```python
from build123d import *

# Parameters (mm, degrees)
SKETCH1_R           = 12.0269
BOSS_EXTRUDE1_DEPTH = 3.03784
BOSS_EXTRUDE2_DEPTH = 5.0038
FILLET1_R           = 5.08
FILLET2_R           = 0.381


with BuildPart() as part:
    # Sketch1 → Boss-Extrude1 (new body)
    with BuildSketch(Plane(origin=(0, 0, 0), x_dir=(1, 0, 0), z_dir=(0, 1, 0))):
        with Locations(Location((0, 0, 0), (0, 0, 270))):
            Circle(SKETCH1_R)
        with BuildLine():
            Line((-3.334475635, 5.1562), (3.334475635, 5.1562))
            ThreePointArc((3.334475635, 5.1562), (6.14045, 0), (3.334475635, -5.1562))
            Line((3.334475635, -5.1562), (-3.334475635, -5.1562))
            ThreePointArc((-3.334475635, -5.1562), (-6.14045, 0), (-3.334475635, 5.1562))
        make_face(mode=Mode.SUBTRACT)
    extrude(amount=BOSS_EXTRUDE1_DEPTH)

    # Sketch3 → Boss-Extrude2 (add, symmetric)
    with BuildSketch(Plane.XY):
        Polygon((-6.14045, 3.03784), (-13.285214528, 3.03784), (-17.255205114, -0.932150585), (-15.10712785, -3.08022785), (-12.0269, 0), (-6.14045, 0), align=None)
    extrude(amount=BOSS_EXTRUDE2_DEPTH, both=True)

    # Fillet1
    fillet1_edges = [part.edges().sort_by_distance(p)[0] for p in [
        (-13.285214528, 3.03784, 0),
    ]]
    fillet(fillet1_edges, radius=FILLET1_R)

    # Fillet2
    fillet2_edges = [part.edges().sort_by_distance(p)[0] for p in [
        (6.14045, 3.03784, 0),
        (0, 3.03784, -5.1562),
        (12.0269, 3.03784, 0),
        (-10.936558379, 1.51892, -5.0038),
        (-10.936558379, 1.51892, 5.0038),
        (-11.058784005, 3.03784, 5.0038),
        (-16.181166482, -2.006189217, 5.0038),
        (-11.058784005, 3.03784, -5.0038),
        (-16.181166482, -2.006189217, -5.0038),
        (-17.255205114, -0.932150585, 0),
        (-16.014158597, 0.308895932, -5.0038),
        (-16.014158597, 0.308895932, 5.0038),
        (-13.125041468, 2.651148025, -5.0038),
        (-13.125041468, 2.651148025, 5.0038),
        (-6.14045, 3.03784, 0),
        (0, 3.03784, 5.1562),
    ]]
    fillet(fillet2_edges, radius=FILLET2_R)


solid = part.part
```
Read the model definition and answer for the solid it produces. Units are mm, in the model's axes. A direction names the side the tool comes from. Give positions to 0.01 mm unless a question says otherwise; leave off trailing zeros. Write each loop counter-clockwise with the first axis right and the second up, starting at its lowest first coordinate (ties: lowest second). Pieces come first, ordered by that corner, then holes. Notation, with made-up numbers: (-5.5, 32) -> (24.5, 32) arc R21 ccw to (24.5, 36) -> close; hole circle Ø5 at (51.5, 37). An arc over 180 degrees is marked (long way). Answer in a Markdown table with one row per item.
1) Determine the mould class of faces 6 (the cylindrical face through (-6.14, 1.31, 0.09)), 7 (the flat face through (-13.589, -1.562, 0.07)), 8 (the cylindrical face through (-15.82, 0.35, -4.89)) for opening direction Z: released by +Z, released by -Z, zero draft, split by the parting line, or undercut.
Results list:
| item | result |
|---|---|
| face 6 | undercut |
| face 7 | zero draft |
| face 8 | released by -Z |
2) Straight lines are drawn through the part: line 1 (Y direction, x = 3.5, z = -8); line 2 (Z direction, x = -14.25, y = -1); line 3 (X direction, y = 1.5, z = -0.5). For each, find the intervals that lie inside material, in ascending order. Write a range as [from, to].
Results list:
| item | result |
|---|---|
| line 1 | [0, 3.04] |
| line 2 | [-5, 5] |
| line 3 | [-14.82, -6.12], [6.12, 12.02] |
3) Each of these flat-tipped pins is pushed along its axis until it touches: pin 1 Ø1.5 at (y, z) = (1, -7) entering from +X; pin 2 Ø8 at (x, z) = (-2.5, -2.5) entering from +Y; pin 3 Ø6 at (x, z) = (-8, 1) entering from -Y; pin 4 Ø1.5 at (y, z) = (-2, -3.5) entering from -X. Where does it stop, or does it pass through?
Results list:
| item | result |
|---|---|
| pin 1 | x = 10.28 |
| pin 2 | y = 3.04 |
| pin 3 | y = 0 |
| pin 4 | x = -16.94 |
4) Section B-B on z = 0 is taken. Give the vertices of the cut face in (x, y), plus the area to 3 significant figures.
Results list:
| item | result |
|---|---|
| outline | (-16.99, -1.2) -> (-15.11, -3.08) -> (-12.03, 0) -> (-6.14, 0) -> (-6.14, 2.66) arc R0.38 ccw to (-6.52, 3.04) -> (-11.18, 3.04) arc R5.08 ccw to (-14.77, 1.55) -> (-16.99, -0.66) arc R0.38 ccw to start; (6.14, 0) -> (12.03, 0) -> (12.03, 2.66) arc R0.38 ccw to (11.65, 3.04) -> (6.52, 3.04) arc R0.38 ccw to (6.14, 2.66) -> close |
| area | 52.1 mm^2 |
5) Section A-A on x = 0 is taken. Give the vertices of the cut face in (y, z), plus the area to 3 significant figures.
Results list:
| item | result |
|---|---|
| outline | (0, -12.03) -> (2.66, -12.03) arc R0.38 ccw to (3.04, -11.65) -> (3.04, -5.54) arc R0.38 ccw to (2.66, -5.16) -> (0, -5.16) -> close; (0, 5.16) -> (2.66, 5.16) arc R0.38 ccw to (3.04, 5.54) -> (3.04, 11.65) arc R0.38 ccw to (2.66, 12.03) -> (0, 12.03) -> close |
| area | 41.6 mm^2 |
6) A tool of negligible diameter and unlimited length cuts with its end or side. For faces 1 (the flat face through (-13, 0, -5.004)), 2 (the cylindrical face through (6.14, 1.31, -0.09)), 3 (the flat face through (-13, 0, 5.004)), 4 (the flat face through (0, 0, -6)), 5 (the flat face through (-5, 3.038, 5)), from which of +Z, -Z, +X, -X, +Y, -Y can it reach the whole face along a straight path? Write none if from no direction.
Results list:
| item | result |
|---|---|
| face 1 | -Z, -X, +Y, -Y |
| face 2 | +Y, -Y |
| face 3 | +Z, -X, +Y, -Y |
| face 4 | +Z, -Z, +X, -Y |
| face 5 | +Z, -Z, +X, -X, +Y |
